Part model, mm, in its own coordinate system. Round coordinates to 2 decimals unless told otherwise and drop trailing zeros. Loops run counter-clockwise (first coordinate to the right, second up) from the corner with the lowest first, then second, coordinate; pieces in that order, holes last. Notation, with made-up numbers: M 8,-37 L 67,-37 A9 cw 67,-22 Z; hole C -7,89 d5. An arc over 180 degrees is marked long. Write each question's results on one line, items separated by ' | '.
Autodesk Inventor part; units mm, degrees
ref_plane "YZ Plane" through (0, 0, 0) normal (1, 0, 0) x (0, 1, 0)
ref_plane "XZ Plane" through (0, 0, 0) normal (0, 1, 0) x (-1, 0, 0)
ref_plane "XY Plane" through (0, 0, 0) normal (0, 0, 1) x (1, 0, 0)
sketch "Sketch1" plane through (0, 0, 0) normal (0, 1, 0) x (-1, 0, 0)
  line L0 (4.5242, 7.5266) -> (-15.9758, 7.5266)
  line L1 (-15.9758, 7.5266) -> (-15.9758, -12.9734)
  line L2 (-15.9758, -12.9734) -> (4.5242, -12.9734)
  line L3 (4.5242, -12.9734) -> (4.5242, 7.5266)
  circle A0 centre (-5.7258, -2.7234) radius 8
  point P0 (0, 0)
  dimension "d0" = 20.5
  dimension "d1" = 20.5
  dimension "d2" = 16
extrude "Extrusion1" add sketch "Sketch1" along normal blind 5
sketch "Sketch2" plane through (-4.5242, 0, -12.9734) normal (-1, 0, 0) x (0, 0, 1)
  line L0 (20.5, 0) -> (25.5, 0)
  line L1 (20.5, 0) -> (20.5, 5)
  line L2 (25.5, 0) -> (20.5, 5)
  line L3 (0, 0) -> (-5, 0)
  line L4 (-5, 0) -> (0, 5)
  line L5 (0, 0) -> (0, 5)
  line L6 (0, 5) -> (0, 0)
  point P0 (12.9734, 0)
  dimension "d6" = 5
  dimension "d7" = 5
extrude "Extrusion2" add sketch "Sketch2" against normal up to surface (20.5 mm away)
sketch "Sketch3" plane through (15.9758, 0, 12.5266) normal (1, 0, 0) x (0, 0, -1)
  point P0 (12.5266, 0)
sketch "Sketch4" plane through (-4.5242, 0, -17.9734) normal (-1, 0, 0) x (0, 0, 1)
  line L0 (0, 0) -> (30.5, 0)
  line L1 (30.5, 0) -> (25.5, 5)
  line L2 (5, 5) -> (25.5, 5)
  line L3 (5, 5) -> (0, 0)
  point P0 (17.9734, 0)
extrude "Extrusion3" add sketch "Sketch4" along normal blind 3.5
sketch "Sketch5" plane through (15.9758, 0, 12.5266) normal (1, 0, 0) x (0, 0, -1)
  line L0 (0, 0) -> (30.5, 0)
  line L1 (25.5, 5) -> (30.5, 0)
  line L2 (5, 5) -> (25.5, 5)
  line L3 (0, 0) -> (5, 5)
  line L4 (4.9586, 5.1) -> (25.5414, 5.1)
  line L5 (25.5414, 5.1) -> (30.7414, -0.1)
  line L6 (30.7414, -0.1) -> (-0.2414, -0.1)
  line L7 (-0.2414, -0.1) -> (4.9586, 5.1)
  line L8 (25.5, 5) -> (25.6414, 5)
  line L9 (30.5, 0) -> (30.6414, 0)
  line L10 (0, 0) -> (-0.1414, 0)
  line L11 (5, 5) -> (4.8586, 5)
  point P0 (12.5266, 0)
  dimension "d12" = 0.1
extrude "Extrusion4" add sketch "Sketch5" against normal up to surface (24 mm away) contours L10 L7 L11 L3 | L1 L8 L5 L9
properties part number "bearing_bed_arm2_tight"
Item 1: Wall check: L1, parallel to X at y = 3.1, z = 0.5; L2, parallel to X at y = 3.4, z = -4; L3, parallel to Z at x = 11.5, y = 4.55. Give the ranges that are in metal, low to high.
Filled sheet:
L1: -8.02 to -1.6, 13.05 to 15.98 | L2: -8.02 to -2.17, 13.62 to 15.98 | L3: -13.56 to -8.26, 2.81 to 8.12
Item 2: Band-saw the part on D-D on x = -3. Give the cut face in (y, z), and give its area (3 significant figures).
Filled sheet:
outline: M 0,-18.11 L 5,-13.11 L 5,7.67 L 0,12.67 Z | area: 129 mm^2
Item 3: Band-saw the part on B-B on x = 12.5. Give the cut face in (y, z).
Filled sheet:
outline: M 0,-18.11 L 5,-13.11 L 5,-6.98 L 0,-6.98 Z; M 0,1.53 L 5,1.53 L 5,7.67 L 0,12.67 Z
Item 4: Band-saw the part on C-C on y = 0.55. Give the cut face in (x, z).
Filled sheet:
outline: M -8.02,-17.56 L 15.98,-17.56 L 15.98,12.12 L -8.02,12.12 Z; hole C 5.73,-2.72 d16
Item 5: Two-plate mould, pull along Z, no slides. Class faces 1 (the flat face through (15.976, 2, -3)), 2 (the cylindrical face through (-1.905, 2.465, -5.126)), 3 (the flat face through (4.144, 2.535, -15.58)): +Z half, -Z half, draft (parallel to the pull), parting line (faces both ways), or undercut.
Filled sheet:
face 1: draft | face 2: undercut | face 3: -Z half
Item 6: Band-saw the part on A-A on z = 4.5. Give the cut face in (x, y).
Filled sheet:
outline: M -8.02,0 L 2.29,0 L 2.29,5 L -8.02,5 Z; M 9.16,0 L 15.98,0 L 15.98,5 L 9.16,5 Z
